Input: dimensioned drawing with shaded views. Units: mm. Origin: part minimum x, y, z. Coordinates: 2 decimals unless noted, no trailing zeros. Order: outer loops, then holes, each group sorted by start corner. A loop starts at its lowest first (then second) coordinate and runs counter-clockwise, first axis right, second up. Notation, with made-up numbers: (22.25, 62) -> (35.25, 62) arc R18 cw to (35.25, 77) -> close; hole circle Ø5 at (86, 25). An arc over 180 degrees is marked (long way). Put each result on its own line as item: value.
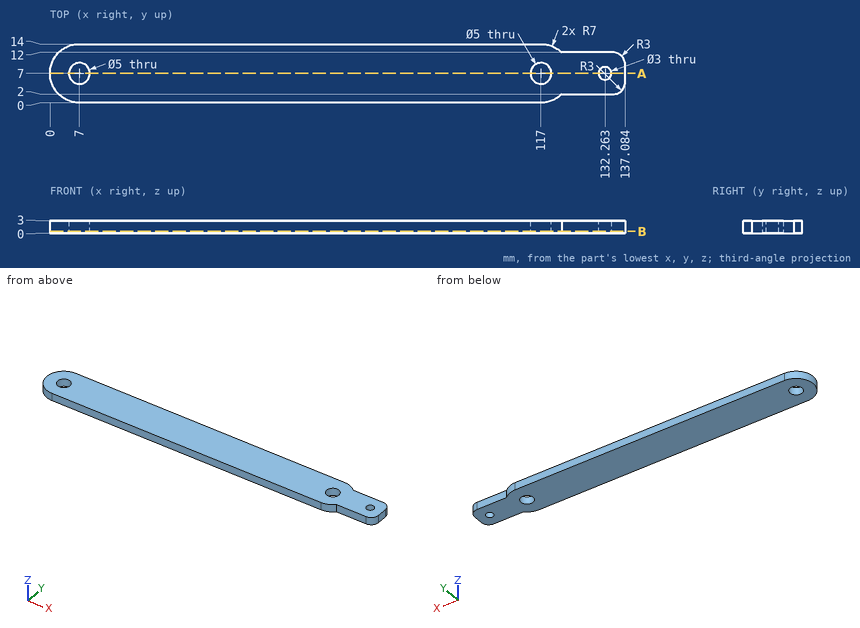
1. Cut plane B-B on z = 0.45. Output: boundary loops of the cut face in (x, y) (1 decimal).
Numbers:
outline: (7, 0) -> (117, 0) arc R7 ccw to (121.9, 2) -> (134.1, 2) arc R3 ccw to (137.1, 5) -> (137.1, 9) arc R3 ccw to (134.1, 12) -> (121.9, 12) arc R7 ccw to (117, 14) -> (7, 14) arc R7 ccw to start; hole circle Ø5 at (7, 7); hole circle Ø5 at (117, 7); hole circle Ø3 at (132.3, 7)
2. Cut plane A-A on y = 7. Output: boundary loops of the cut face in (x, z) (1 decimal).
Numbers:
outline: (0, 0) -> (4.5, 0) -> (4.5, 3) -> (0, 3) -> close; (9.5, 0) -> (114.5, 0) -> (114.5, 3) -> (9.5, 3) -> close; (119.5, 0) -> (130.8, 0) -> (130.8, 3) -> (119.5, 3) -> close; (133.8, 0) -> (137.1, 0) -> (137.1, 3) -> (133.8, 3) -> close
3. First-contact query: pin 1 (1.5 mm diameter, centred on x = 127, z = 1.5, fed in from -Y). Flat tip, straight axial feed; report the tip coordinate or a pass-through.
Numbers:
pin 1: stops at y = 2
4. Ray query, line 1 along X through (y, z) = (7, 1.75) (1 decimal); line 2 along X through (y, z) = (6.75, 2.6) (1 decimal); line 3 along Y through (x, z) = (7, 0.85). Return the intervals inside material, ascending.
Numbers:
line 1: x = 0 to 4.5, 9.5 to 114.5, 119.5 to 130.8, 133.8 to 137.1
line 2: x = 0 to 4.5, 9.5 to 114.5, 119.5 to 130.8, 133.7 to 137.1
line 3: y = 0 to 4.5, 9.5 to 14
